from build123d import *


with BuildPart() as part:
    # Sketch15 → Revolve4 (revolve)
    with BuildSketch(Plane.XY, mode=Mode.PRIVATE) as revolve4_sk:
        with BuildLine():
            Line((-3.175, -2.38125), (-3.175, 2.38125))
            Line((-3.175, 2.38125), (-5.788733992, 2.38125))
            ThreePointArc((-5.788733992, 2.38125), (-6.185608992, 2.216858992), (-6.35, 1.819983992))
            Line((-6.35, 1.819983992), (-6.35, 0.79375))
            Line((-6.35, 0.79375), (-4.7625, 0.79375))
            Line((-4.7625, 0.79375), (-4.7625, -0.79375))
            Line((-4.7625, -0.79375), (-6.35, -0.79375))
            Line((-6.35, -0.79375), (-6.35, -1.819983992))
            ThreePointArc((-6.35, -1.819983992), (-6.185608992, -2.216858992), (-5.788733992, -2.38125))
            Line((-5.788733992, -2.38125), (-3.175, -2.38125))
        make_face()
    revolve(revolve4_sk.sketch.rotate(Axis((0, -2.38125, 0), (0, 1, 0)), 90), axis=Axis((0, -2.38125, 0), (0, 1, 0)))


solid = part.part
Can you work these out from the model? Positions are in its coordinate system, mm. A direction names the side the tool comes from. Coordinates: 2 decimals unless noted, no trailing zeros. Write each loop counter-clockwise with the first axis right and the second up, starting at its lowest first coordinate (ties: lowest second). Pieces come first, ordered by that corner, then holes. Notation, with made-up numbers: (-27, -22) - (-16, -22) arc R33 cw to (-16, 12) - close; hole circle Ø2 at (6.25, 42). An arc over 180 degrees is marked (long way). Return JSON: item names as keys, results as strings. Group by question number.
Item 1: Please list where these lines run through material, in increasing order: probe 1 along X at (y, z) = (-0.4, 0) (1 decimal); probe 2 along Y at (x, z) = (4, -3.5); probe 3 along X at (y, z) = (1.35, 0) (3 decimals).
Item 2: If we section it at D-D (y = 2.1): Write out the boundary of the cut face in (x, z) (3 decimals), then the cut area to 3 significant figures.
Item 3: We'd pull the mould along Y, two halves only. Please class faces 3 (the face through (-2.5, 2.381, -2.5)), 4 (the face through (-4.65, -0.01, -1.03)), 5 (the face through (-3.86, -1.31, -5.04)): pulls with the +Y half, pulls with the -Y half, needs draft (parallel to the pull), parting line crosses it, or undercut.
Item 4: If we section it at C-C (y = 1.3): Write out the boundary of the cut face in (x, z) (3 decimals), then the cut area to 3 significant figures.
Item 5: Which directions (+Z, -Z, +X, -X, +Y, -Y) give clear straight access to the entire face, cutting with the end or side of a thin tool? Please do faces 1 (the face through (-1.93, 0.03, -2.52)), 2 (the face through (5, -0.794, -1)).
Item 6: I'm going to push flat-ended pins straight in: pin 1 Ø1 at (x, z) = (4.5, 4.5) entering from -Y; pin 2 Ø1 at (y, z) = (-1.5, -2.5) entering from +X. Where does each tip first touch, or does it pass through?
Return value:
{
 "1": {"probe 1": "x = -4.8 to -3.2, 3.2 to 4.8", "probe 2": "y = -2.38 to -0.79, 0.79 to 2.38", "probe 3": "x = -6.35 to -3.175, 3.175 to 6.35"},
 "2": {"outline": "circle Ø12.55 at (0, 0); hole circle Ø6.35 at (0, 0)", "area": "92.0 mm^2"},
 "3": {"face 3": "pulls with the +Y half", "face 4": "undercut", "face 5": "needs draft"},
 "4": {"outline": "circle Ø12.7 at (0, 0); hole circle Ø6.35 at (0, 0)", "area": "95.0 mm^2"},
 "5": {"face 1": "+Y, -Y", "face 2": "none"},
 "6": {"pin 1": "stops at y = -2.38", "pin 2": "stops at x = 6.03"}
}
